Can you work these out from the drawing? Everything is in mm from the part's minimum corner. A direction names the side the tool comes from. Give positions to 0.01 mm unless a question says otherwise; leave off trailing zeros. Write each loop counter-clockwise with the first axis right and the second up, starting at its lowest first coordinate (ties: lowest second). Pieces come first, ordered by that corner, then holes. Notation, with made-up numbers: (-29, -30.75) -> (30, -30.75) arc R5 ccw to (30, -26.75) -> close; hole circle Ø5 at (58.25, 22). An arc over 180 degrees is marked (long way). Use one line per item in the form item = value.
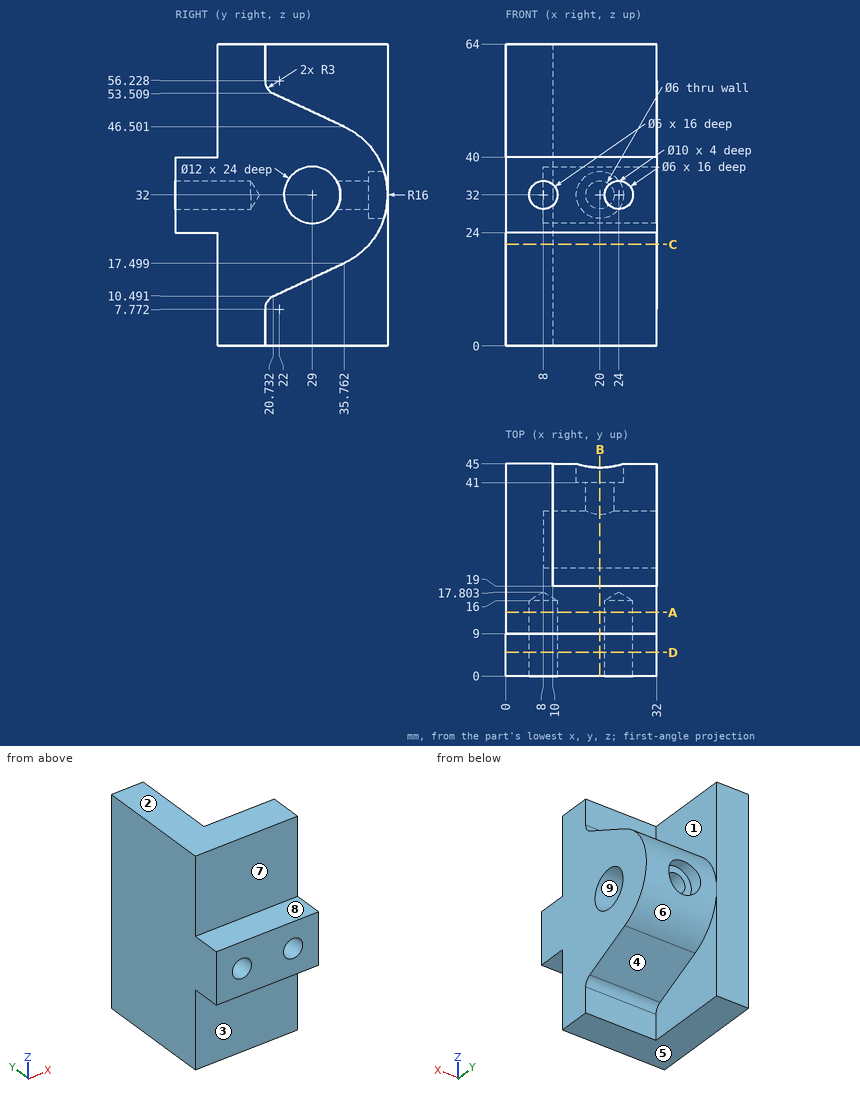
Q1. If I drill on line 1 along Z through (x, y) = (8, 12); line 2 along X through (y, z) = (7, 32); line 3 along Z through (x, y) = (8, 7.5), over which ranges is the centre line in solid material (lowest first)? Write a range as from..to.
Result set:
line_1 = 0..29, 35..64
line_2 = 0..5, 11..21, 27..32
line_3 = 24..29, 35..40
Q2. I want a section at C-C, the plane z = 21.5. Write out the boundary of the cut face in (x, y).
Result set:
outline = (0, 9) -> (32, 9) -> (32, 41.07) -> (10, 41.07) -> (10, 45) -> (0, 45) -> close
Q3. If we mould it in two halves opening along Z, with no side actions, what happens to the marked faces 6, 7, 8 and 9? For each: +Z half, -Z half, draft (parallel to the pull), parting line (faces both ways), or undercut.
Result set:
face_6 = parting line
face_7 = draft
face_8 = +Z half
face_9 = undercut
Q4. I want a section at D-D, the plane y = 5. Write out the boundary of the cut face in (x, z).
Result set:
outline = (0, 24) -> (32, 24) -> (32, 40) -> (0, 40) -> close; hole circle Ø6 at (8, 32); hole circle Ø6 at (24, 32)
Q5. Which directions (+Z, -Z, +X, -X, +Y, -Y) give clear straight access to the entire face, cutting with the end or side of a thin tool? Please do the marked faces 1, 2, 3, 4 and 5.
Result set:
face_1 = +Z, +X, +Y
face_2 = +Z, +X, -X, +Y, -Y
face_3 = -Z, +X, -X, -Y
face_4 = -Z, +X, +Y
face_5 = -Z, +X, -X, +Y, -Y
Q6. I want a section at B-B, the plane x = 20. Write out the boundary of the cut face in (y, z), and give its area (3 significant figures).
Result set:
outline = (0, 24) -> (9, 24) -> (9, 0) -> (19, 0) -> (19, 7.77) arc R3 cw to (20.73, 10.49) -> (35.76, 17.5) arc R16 ccw to (44.2, 27) -> (41, 27) -> (41, 29) -> (34.2, 29) arc R6 cw (long way) to (34.2, 35) -> (41, 35) -> (41, 37) -> (44.2, 37) arc R16 ccw to (35.76, 46.5) -> (20.73, 53.51) arc R3 cw to (19, 56.23) -> (19, 64) -> (9, 64) -> (9, 40) -> (0, 40) -> close
area = 1,410 mm2
Q7. I want a section at A-A, the plane y = 13.5. Write out the boundary of the cut face in (x, z), and give its area (3 significant figures).
Result set:
outline = (0, 0) -> (32, 0) -> (32, 64) -> (0, 64) -> close; hole circle Ø6 at (8, 32); hole circle Ø6 at (24, 32)
area = 1,990 mm2
Q8. Will these pins go through, and if not, where does the flat tip stop? pin 1 Ø2.5 at (x, z) = (24, 5.5) entering from +Y; pin 2 Ø1 at (x, y) = (24.5, 31.5) entering from -Z; pin 3 Ø3 at (x, z) = (21, 19.5) entering from -Y.
Result set:
pin_1 = 19
pin_2 = 15.28
pin_3 = 9
